Autodesk Inventor part; units mm, degrees
ref_plane "YZ Plane" through (0, 0, 0) normal (1, 0, 0) x (0, 1, 0)
ref_plane "XZ Plane" through (0, 0, 0) normal (0, 1, 0) x (-1, 0, 0)
ref_plane "XY Plane" through (0, 0, 0) normal (0, 0, 1) x (1, 0, 0)
sketch "Sketch1" plane through (0, 0, 0) normal (0, 0, 1) x (1, 0, 0)
  line L0 (3.9408, -0.7944) -> (3.5592, -0.7944)
  line L1 (1.4408, -0.7944) -> (1.0592, -0.7944)
  line L2 (-1.0592, -0.7944) -> (-1.4408, -0.7944)
  line L3 (-3.5592, -0.7944) -> (-3.9408, -0.7944)
  line L4 (-6.0592, -0.7944) -> (-6.25, -0.7944)
  line L5 (6.25, -0.7944) -> (6.0592, -0.7944)
  line L6 (6.25, -0.7944) -> (6.25, -8.7944)
  line L7 (6.25, -8.7944) -> (-6.25, -8.7944)
  line L8 (-6.25, -8.7944) -> (-6.25, -0.7944)
  line L9 (-6.25, -0.7944) -> (-6.0592, -0.7944)
  line L10 (-3.9408, -0.7944) -> (-3.5592, -0.7944)
  line L11 (-1.4408, -0.7944) -> (-1.0592, -0.7944)
  line L12 (1.0592, -0.7944) -> (1.4408, -0.7944)
  line L13 (3.5592, -0.7944) -> (3.9408, -0.7944)
  line L14 (6.0592, -0.7944) -> (6.25, -0.7944)
  line L15 (-6.25, -0.7944) -> (6.25, -0.7944)
  point P0 (0, 0)
  dimension "height" = 8
extrude "Extrusion1" add sketch "Sketch1" against normal blind 15
hole "Hole1" at (-0.125, -8.7944, -2.5) direction (0, 1, 0) diameter 2.459 end through all
hole "Hole2" at (6.25, -4.7944, -7.5) direction (-1, 0, 0) diameter 3.242 end through all
sketch "Sketch2" plane through (0, 0, -15) normal (0, 0, -1) x (-1, 0, 0)
  line L0 (-6.25, -0.7944) -> (-6.25, -8.7944)
  line L1 (-6.25, -8.7944) -> (6.25, -8.7944)
  line L2 (6.25, -8.7944) -> (6.25, -0.7944)
  line L3 (6.25, -0.7944) -> (-6.25, -0.7944)
  point P0 (0, 0)
extrude "Extrusion4" add sketch "Sketch2" along normal blind 10
sketch "Sketch4" plane through (-6.25, -8.7944, 0) normal (-1, 0, 0) x (0, 0, 1)
  line L0 (-25, 0) -> (-20, 0)
  line L1 (-20, 0) -> (-20, 8)
  line L2 (-20, 8) -> (-25, 8)
  line L3 (-25, 8) -> (-25, 0)
  point P0 (0, 8.7944)
  dimension "d28" = 5
  dimension "d40" = 8
extrude "Extrusion5" add sketch "Sketch4" along normal blind 10
hole "Hole3" at (-11.25, -4.7944, -20) direction (0, 0, -1) diameter 2.459 end through all countersink diameter 6 countersink angle 90
pattern_linear "Rectangular Pattern1" count 2 spacing 22.5 along (1, 0, 0) of "Extrusion5", "Hole3"
equation "\"d12\" = 0.5 * width"
equation "\"d13\" = 0.5 * height"
properties part number "T2.5 belt holder fixed" material "Aluminum 6061"
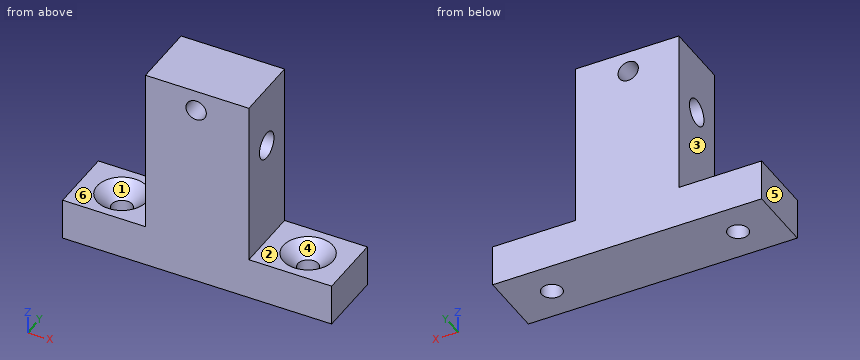
Geometry check sheet. Reference: the model listing, model coordinates, mm. Face numbers are marked on the shaded views. A direction names the side the tool comes from. Give positions to 0.01 mm unless a question says otherwise; leave off trailing zeros. Loops run counter-clockwise (first coordinate to the right, second up) from the corner with the lowest first, then second, coordinate; pieces in that order, holes last. Notation, with made-up numbers: M 84.5,39.5 L 109.5,39.5 A18 ccw 109.5,69.5 Z; hole C 1,68 d6. An arc over 180 degrees is marked long. Answer as a JSON object with one key per item and string values. Group by question number.
Item 1: Sectioned sample at D-D on x = 3. Record the boundary of the cut face in (y, z).
Item 2: Sectioned sample at C-C on z = -7.5. Record the boundary of the cut face in (x, y), plus the area to 3 significant figures.
Item 3: Material ranges on L1, parallel to Y at x = -11.25, z = -22.9; L2, parallel to X at y = -4.75, z = -2.5; L3, parallel to X at y = -5, z = -14.5, recorded low to high.
Item 4: Gauge pin test, flat ends, axial feed: pin 1 (3.5 mm diameter, centred on y = -4.79, z = -7.5, fed in from -X); pin 2 (2 mm diameter, centred on x = -11.25, y = -4.79, fed in from -Z); pin 3 (4 mm diameter, centred on x = 12.5, y = -5.5, fed in from +Z). Record the tip position at first contact, or that the pin passes through.
Item 5: Access from +Z, -Z, +X, -X, +Y, -Y to the whole of each face (thin tool, end or side, straight path). Record for the marked faces 1, 2 and 3.
Item 6: Mould release check, pull along X, two halves, no side actions. Record for the marked faces 4, 5 and 6: pulls with the +X half, pulls with the -X half, needs draft (parallel to the pull), parting line crosses it, or undercut.
Item 7: Sectioned sample at A-A on z = -2.5. Record the boundary of the cut face in (x, y), plus the area to 3 significant figures.
Item 8: Sectioned sample at B-B on x = 11.25. Record the boundary of the cut face in (y, z).
Findings below:
{
 "1": {"outline": "M -8.79,-25 L -0.79,-25 L -0.79,0 L -8.79,0 Z; hole C -4.79,-7.5 d3.24"},
 "2": {"outline": "M -6.25,-8.79 L 6.25,-8.79 L 6.25,-6.42 L -6.25,-6.42 Z; M -6.25,-3.17 L 6.25,-3.17 L 6.25,-0.79 L -6.25,-0.79 Z", "area": "59.5 mm2"},
 "3": {"L1": "-8.79 to -6.02, -3.56 to -0.79", "L2": "-6.25 to -1.35, 1.1 to 6.25", "L3": "-6.25 to 6.25"},
 "4": {"pin 1": "x = -6.25", "pin 2": "through", "pin 3": "z = -20"},
 "5": {"face 1": "+Z", "face 2": "+Z, +X, +Y, -Y", "face 3": "+Z, -X, +Y, -Y"},
 "6": {"face 4": "undercut", "face 5": "pulls with the -X half", "face 6": "needs draft"},
 "7": {"outline": "M -6.25,-8.79 L -1.35,-8.79 L -1.35,-0.79 L -6.25,-0.79 Z; M 1.1,-8.79 L 6.25,-8.79 L 6.25,-0.79 L 1.1,-0.79 Z", "area": "80.3 mm2"},
 "8": {"outline": "M -8.79,-25 L -6.02,-25 L -6.02,-21.77 L -7.79,-20 L -8.79,-20 Z; M -3.56,-25 L -0.79,-25 L -0.79,-20 L -1.79,-20 L -3.56,-21.77 Z"}
}
